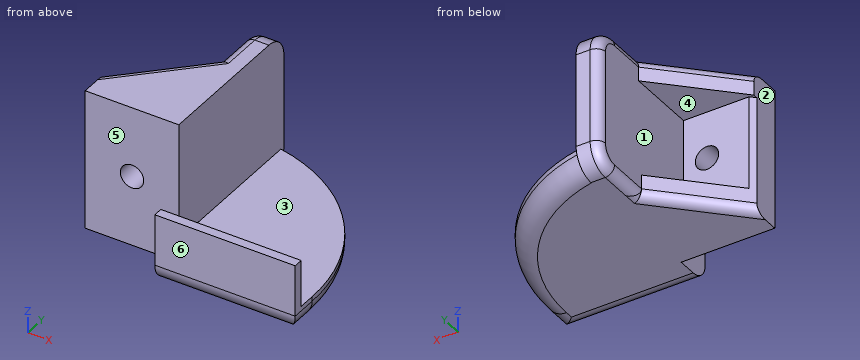
```python
from build123d import *

# Parameters (mm, degrees)
F0_W          = 30
F0_H          = 42
F1_DEPTH      = 5
F2_T1_DEPTH   = 186.6590212458
F3_W          = 30
F3_H          = 2
F4_DEPTH      = 10
F5_W          = 35
F5_H          = 30
F6_DEPTH      = 5
F7_W          = 7
F7_H          = 30
F8_DEPTH      = 15
F9_R          = 2.5
F10_DEPTH     = 10
F11_R         = 4
F12_W         = 15
F12_H         = 14
F13_DEPTH     = 5
F14_W         = 15
F14_H         = 15
F15_DEPTH     = 5
F16_T4_DEPTH  = 35.8601958556
F16_T9_DEPTH  = 35.8601958556
F17_R         = 5
F18_T1_DEPTH  = 20
F18_T6_DEPTH  = 9.5699020722
F18_T11_DEPTH = 31.2132034356
F18_T16_DEPTH = 31.2132034356
F18_T21_DEPTH = 14
F18_T24_ANGLE = 90
F18_T26_ANGLE = 90
F18_T30_DEPTH = 13
F18_T36_DEPTH = 14
F18_T40_DEPTH = 31.2132034356
F18_T47_DEPTH = 13
F18_T51_DEPTH = 31.2132034356


# Not quite as in the source:
# - a fillet or chamfer that OpenCascade refuses, or shapes differently, is made with other operations: its cross-section is extruded or revolved along the edge and cut away or added


with BuildPart() as f1:
    # F0 (on Top) → F1 (new body)
    with BuildSketch(Plane.XY):
        with Locations((15, 21)):
            Rectangle(F0_W, F0_H)
    extrude(amount=F1_DEPTH)

    # F2: fillet of radius 37 on 1 edges, made by hand

    # F2_s2 → F2_t1 (cut)
    with BuildSketch(Plane.XY.offset(-90.8295106229)):
        with BuildLine():
            ThreePointArc((30, 5.6681957508), (21.5306852354, 29.2266337296), (0, 42))
            Line((0, 42), (30, 42))
            Line((30, 42), (30, 5.6681957508))
        make_face()
    extrude(amount=F2_T1_DEPTH, mode=Mode.SUBTRACT)

    # F3 (on face) → F4 (join)
    with BuildSketch(Plane.XY.offset(5)):
        with Locations((15, 1)):
            Rectangle(F3_W, F3_H)
    extrude(amount=F4_DEPTH)

    # F5 (on face) → F6 (join)
    with BuildSketch(Plane(origin=(0, 0, 0), x_dir=(0, -1, 0), z_dir=(-1, 0, 0))):
        with Locations((-25.5, 15)):
            Rectangle(F5_W, F5_H)
    extrude(amount=F6_DEPTH)

    # F7 (on face) → F8 (join)
    with BuildSketch(Plane(origin=(-5, 0, 0), x_dir=(0, -1, 0), z_dir=(-1, 0, 0))):
        with Locations((-11.5, 15)):
            Rectangle(F7_W, F7_H)
    extrude(amount=F8_DEPTH)

    # F9 (on face) → F10 (cut)
    with BuildSketch(Plane(origin=(0, 15, 0), x_dir=(-1, 0, 0), z_dir=(0, 1, 0))):
        with Locations((10, 15)):
            Circle(F9_R)
    extrude(amount=-F10_DEPTH, mode=Mode.SUBTRACT)

    # F11
    f11_edges = [f1.edges().sort_by_distance(p)[0] for p in [
        (21.530685, 29.226634, 0),
        (15, 0, 0),
    ]]
    fillet(f11_edges, radius=F11_R)

    # F12 (on face) → F13 (join)
    with BuildSketch(Plane(origin=(0, 0, 0), x_dir=(1, 0, 0), z_dir=(0, 0, -1))):
        with Locations((-12.5, -22)):
            Rectangle(F12_W, F12_H)
    extrude(amount=-F13_DEPTH)

    # F14 (on face) → F15 (join)
    with BuildSketch(Plane.XY.offset(30)):
        with Locations((-12.5, 22.5)):
            Rectangle(F14_W, F14_H)
    extrude(amount=-F15_DEPTH)

    # F16: chamfer of 15 on 2 edges, made by hand


with BuildPart() as f16_tool2:
    # F16_s3 → F16_t4 (new body)
    with BuildSketch(Plane.XY.offset(45.4300979278)):
        with BuildLine():
            Line((-20.4242640687, 14.5757359313), (-4.5757359313, 30.4242640687))
            Line((-4.5757359313, 30.4242640687), (-4.5757359313, 30.7242640687))
            ThreePointArc((-4.5757359313, 30.7242640687), (-12.2878679656, 30.3), (-20, 30.3))
            Line((-20, 30.3), (-20.3, 30))
            ThreePointArc((-20.3, 30), (-20.3, 22.2878679656), (-20.7242640687, 14.5757359313))
            Line((-20.7242640687, 14.5757359313), (-20.4242640687, 14.5757359313))
        make_face()
    extrude(amount=-F16_T4_DEPTH)

    split(bisect_by=Plane.YZ.offset(-5), keep=Keep.BOTTOM)


with BuildPart() as f1_1:
    add(f1.part)

    # F16_t1: cut F16_tool2
    add(f16_tool2.part, mode=Mode.SUBTRACT)


with BuildPart() as f16_tool7:
    # F16_s8 → F16_t9 (new body)
    with BuildSketch(Plane.XY.offset(-15.4300979278)):
        with BuildLine():
            Line((-4.5757359313, 29.4242640687), (-20.4242640687, 13.5757359313))
            Line((-20.4242640687, 13.5757359313), (-20.7242640687, 13.5757359313))
            ThreePointArc((-20.7242640687, 13.5757359313), (-20.3, 21.2878679656), (-20.3, 29))
            Line((-20.3, 29), (-20, 29.3))
            ThreePointArc((-20, 29.3), (-12.2878679656, 29.3), (-4.5757359313, 29.7242640687))
            Line((-4.5757359313, 29.7242640687), (-4.5757359313, 29.4242640687))
        make_face()
    extrude(amount=F16_T9_DEPTH)

    split(bisect_by=Plane.YZ.offset(-5), keep=Keep.BOTTOM)


with BuildPart() as f1_2:
    add(f1_1.part)

    # F16_t6: cut F16_tool7
    add(f16_tool7.part, mode=Mode.SUBTRACT)

    # F17
    f17_edges = [f1_2.edges().sort_by_distance(p)[0] for p in [
        (-2.5, 43, 0),
        (-2.5, 43, 30),
    ]]
    fillet(f17_edges, radius=F17_R)

    # F18: fillet of radius 2 on 9 edges, made by hand

    # F18_s2 → F18_t1 (cut)
    with BuildSketch(Plane.XY.offset(5)):
        with BuildLine():
            ThreePointArc((-3, 43), (-4.4142135624, 42.4142135624), (-5, 41))
            Line((-5, 41), (-5, 43))
            Line((-5, 43), (-3, 43))
        make_face()
    extrude(amount=F18_T1_DEPTH, mode=Mode.SUBTRACT)


with BuildPart() as f18_tool4:
    # F18_s5 → F18_t6 (new body)
    with BuildSketch(Plane.XY.offset(25)):
        with BuildLine():
            ThreePointArc((-20, 13), (-19.4142135624, 14.4142135624), (-18, 15))
            Line((-18, 15), (-20, 15))
            Line((-20, 15), (-20, 13))
        make_face()
    extrude(amount=-F18_T6_DEPTH)

    split(bisect_by=Plane(origin=(-17, 17, 0), x_dir=(0, 0, 1), z_dir=(-0.7071067812, 0.7071067812, 0)), keep=Keep.TOP)


with BuildPart() as f1_3:
    add(f1_2.part)

    # F18_t3: cut F18_tool4
    add(f18_tool4.part, mode=Mode.SUBTRACT)


with BuildPart() as f18_tool9:
    # F18_s10 → F18_t11 (new body)
    with BuildSketch(Plane(origin=(-6.5355339059, -6.5355339059, 0), x_dir=(0, 0, 1), z_dir=(0.7071067812, 0.7071067812, 0))):
        with BuildLine():
            ThreePointArc((0, -22.0416305603), (0.5857864376, -23.4558441227), (2, -24.0416305603))
            Line((2, -24.0416305603), (0, -24.0416305603))
            Line((0, -24.0416305603), (0, -22.0416305603))
        make_face()
    extrude(amount=F18_T11_DEPTH)

    split(bisect_by=Plane.YZ.offset(-5), keep=Keep.BOTTOM)


with BuildPart() as f1_4:
    add(f1_3.part)

    # F18_t8: cut F18_tool9
    add(f18_tool9.part, mode=Mode.SUBTRACT)


with BuildPart() as f18_tool14:
    # F18_s15 → F18_t16 (new body)
    with BuildSketch(Plane(origin=(16.0355339059, 16.0355339059, 0), x_dir=(0, 0, 1), z_dir=(-0.7071067812, -0.7071067812, 0))):
        with BuildLine():
            ThreePointArc((30, 22.7487373415), (29.4142135624, 24.1629509039), (28, 24.7487373415))
            Line((28, 24.7487373415), (30, 24.7487373415))
            Line((30, 24.7487373415), (30, 22.7487373415))
        make_face()
    extrude(amount=F18_T16_DEPTH)

    split(bisect_by=Plane.YZ.offset(-5), keep=Keep.BOTTOM)


with BuildPart() as f1_5:
    add(f1_4.part)

    # F18_t13: cut F18_tool14
    add(f18_tool14.part, mode=Mode.SUBTRACT)


with BuildPart() as f18_tool19:
    # F18_s20 → F18_t21 (new body)
    with BuildSketch(Plane.XZ.offset(-24)):
        with BuildLine():
            ThreePointArc((-3, 0), (-4.4142135624, 0.5857864376), (-5, 2))
            Line((-5, 2), (-5, 0))
            Line((-5, 0), (-3, 0))
        make_face()
    extrude(amount=-F18_T21_DEPTH)

    split(bisect_by=Plane(origin=(-17, 17, 0), x_dir=(0, 0, 1), z_dir=(-0.7071067812, 0.7071067812, 0)), keep=Keep.TOP)


with BuildPart() as f1_6:
    add(f1_5.part)

    # F18_t18: cut F18_tool19
    add(f18_tool19.part, mode=Mode.SUBTRACT)

    # F18_s23 → F18_t24 (revolve, cut)
    with BuildSketch(Plane.XY.offset(5)):
        with BuildLine():
            ThreePointArc((-3, 43), (-4.4142135624, 42.4142135624), (-5, 41))
            Line((-5, 41), (-5, 43))
            Line((-5, 43), (-3, 43))
        make_face()
    revolve(axis=Axis((-5, 38, 5), (-1, 0, 0)), revolution_arc=F18_T24_ANGLE, mode=Mode.SUBTRACT)

    # F18_s25 → F18_t26 (revolve, cut)
    with BuildSketch(Plane.XY.offset(25)):
        with BuildLine():
            ThreePointArc((-3, 43), (-4.4142135624, 42.4142135624), (-5, 41))
            Line((-5, 41), (-5, 43))
            Line((-5, 43), (-3, 43))
        make_face()
    revolve(axis=Axis((-5, 38, 25), (1, 0, 0)), revolution_arc=F18_T26_ANGLE, mode=Mode.SUBTRACT)


with BuildPart() as f18_tool28:
    # F18_s29 → F18_t30 (new body)
    with BuildSketch(Plane.XZ.offset(-25)):
        with BuildLine():
            ThreePointArc((-3, 30), (-4.4142135624, 29.4142135624), (-5, 28))
            Line((-5, 28), (-5, 30))
            Line((-5, 30), (-3, 30))
        make_face()
    extrude(amount=-F18_T30_DEPTH)

    split(bisect_by=Plane(origin=(-17.5, 17.5, 0), x_dir=(0, 0, 1), z_dir=(-0.7071067812, 0.7071067812, 0)), keep=Keep.TOP)


with BuildPart() as f1_7:
    add(f1_6.part)

    # F18_t27: cut F18_tool28
    add(f18_tool28.part, mode=Mode.SUBTRACT)


with BuildPart() as f18_tool34:
    # F18_s35 → F18_t36 (new body)
    with BuildSketch(Plane.XZ.offset(-24)):
        with BuildLine():
            ThreePointArc((-3, 0), (-4.4142135624, 0.5857864376), (-5, 2))
            Line((-5, 2), (-5, 0))
            Line((-5, 0), (-3, 0))
        make_face()
    extrude(amount=-F18_T36_DEPTH)

    split(bisect_by=Plane(origin=(-17, 17, 0), x_dir=(0, 0, 1), z_dir=(0.7071067812, -0.7071067812, 0)), keep=Keep.TOP)


with BuildPart() as f18_tool38:
    # F18_s39 → F18_t40 (new body)
    with BuildSketch(Plane(origin=(-6.5355339059, -6.5355339059, 0), x_dir=(0, 0, 1), z_dir=(0.7071067812, 0.7071067812, 0))):
        with BuildLine():
            ThreePointArc((0, -22.0416305603), (0.5857864376, -23.4558441227), (2, -24.0416305603))
            Line((2, -24.0416305603), (0, -24.0416305603))
            Line((0, -24.0416305603), (0, -22.0416305603))
        make_face()
    extrude(amount=F18_T40_DEPTH)

    split(bisect_by=Plane.YZ.offset(-5), keep=Keep.TOP)


with BuildPart() as f18_tool34_1:
    add(f18_tool34.part)

    # F18_t42: intersect F18_tool38
    add(f18_tool38.part, mode=Mode.INTERSECT)


with BuildPart() as f1_8:
    add(f1_7.part)

    # F18_t32: cut F18_tool34
    add(f18_tool34_1.part, mode=Mode.SUBTRACT)


with BuildPart() as f18_tool45:
    # F18_s46 → F18_t47 (new body)
    with BuildSketch(Plane.XZ.offset(-25)):
        with BuildLine():
            ThreePointArc((-3, 30), (-4.4142135624, 29.4142135624), (-5, 28))
            Line((-5, 28), (-5, 30))
            Line((-5, 30), (-3, 30))
        make_face()
    extrude(amount=-F18_T47_DEPTH)

    split(bisect_by=Plane(origin=(-17.5, 17.5, 0), x_dir=(0, 0, 1), z_dir=(0.7071067812, -0.7071067812, 0)), keep=Keep.TOP)


with BuildPart() as f18_tool49:
    # F18_s50 → F18_t51 (new body)
    with BuildSketch(Plane(origin=(16.0355339059, 16.0355339059, 0), x_dir=(0, 0, 1), z_dir=(-0.7071067812, -0.7071067812, 0))):
        with BuildLine():
            ThreePointArc((30, 22.7487373415), (29.4142135624, 24.1629509039), (28, 24.7487373415))
            Line((28, 24.7487373415), (30, 24.7487373415))
            Line((30, 24.7487373415), (30, 22.7487373415))
        make_face()
    extrude(amount=F18_T51_DEPTH)

    split(bisect_by=Plane.YZ.offset(-5), keep=Keep.TOP)


with BuildPart() as f18_tool45_1:
    add(f18_tool45.part)

    # F18_t53: intersect F18_tool49
    add(f18_tool49.part, mode=Mode.INTERSECT)


with BuildPart() as f1_9:
    add(f1_8.part)

    # F18_t43: cut F18_tool45
    add(f18_tool45_1.part, mode=Mode.SUBTRACT)


solid = f1_9.part
```
Read the model definition and answer for the solid it produces. Units are mm, in the model's axes. Face numbers are marked on the shaded views. A direction names the side the tool comes from. Round coordinates to 2 decimals unless told otherwise and drop trailing zeros. Write each loop counter-clockwise with the first axis right and the second up, starting at its lowest first coordinate (ties: lowest second). Pieces come first, ordered by that corner, then holes. Notation, with made-up numbers: (44, 71.5) -> (57, 71.5) arc R20 cw to (57, 93.5) -> close; hole circle Ø11 at (67, 71). An arc over 180 degrees is marked (long way). Answer in a Markdown table with one row per item. Add a question column.
1) Determine the mould class of the marked faces 1, 2 and 3 for opening direction Z: pulls with the +Z half, pulls with the -Z half, needs draft (parallel to the pull), parting line crosses it, or undercut.
2) Find section B-B, the plane z = 16.5. Determine the outline of the cut face in (x, y), and give its area (3 significant figures).
3) Which of the six approach directions +Z, -Z, +X, -X, +Y, -Y give full straight-line access (tool end or side, diameter ignored) to the marked faces 4, 5 and 6?
4) Consider line 1 (Z direction, x = -10, y = 12.5); line 2 (Z direction, x = 11.5, y = 22); line 3 (Y direction, x = 14, z = 7.5). Determine where each line is inside the solid, lowest interval first.
5) Find section A-A, the plane z = 6.5. Determine the outline of the cut face in (x, y).
6) Given P1, Ø9, axis at x = 7.5, y = 22, coming from the +Z side; P2, Ø10, axis at x = -15, z = 21, coming from the -Y side; P3, Ø8, axis at y = 37, z = 10, coming from the +X side; P4, Ø8, axis at x = 2, z = 19, coming from the +Y side, each flat-ended and moving along its own axis, determine where each tip first touches the part or whether it passes through.
Findings below:
| question | item | result |
|---|---|---|
| 1 | face 1 | undercut |
| 1 | face 2 | needs draft |
| 1 | face 3 | pulls with the +Z half |
| 2 | outline | (-20, 8) -> (-12, 8) -> (-12, 15) -> (-19, 15) -> (-20, 14) -> close; (-8, 8) -> (0, 8) -> (0, 43) -> (-3, 43) arc R2 ccw to (-5, 41) -> (-5, 15) -> (-8, 15) -> close |
| 2 | area | 251 mm² |
| 3 | face 4 | -X, +Y |
| 3 | face 5 | +Z, -Z, -X, -Y |
| 3 | face 6 | +Z, -Z, +X, -X, -Y |
| 4 | line 1 | 0 to 12.5, 17.5 to 30 |
| 4 | line 2 | 0 to 5 |
| 4 | line 3 | 0 to 2 |
| 5 | outline | (-20, 8) -> (0, 8) -> (0, 43) -> (-3, 43) arc R2 ccw to (-5, 41) -> (-5, 15) -> (-19, 15) -> (-20, 14) -> close; (0, 0) -> (30, 0) -> (30, 2) -> (0, 2) -> close |
| 6 | P1 | z = 5 |
| 6 | P2 | y = 8 |
| 6 | P3 | x = 0 |
| 6 | P4 | y = 43 |
